Geometry check sheet. Reference: the model listing, model coordinates, mm. A direction names the side the tool comes from. Round coordinates to 2 decimals unless told otherwise and drop trailing zeros. Write each loop counter-clockwise with the first axis right and the second up, starting at its lowest first coordinate (ties: lowest second). Pieces come first, ordered by that corner, then holes. Notation, with made-up numbers: M 25,0.5 L 71,0.5 A14 ccw 71,25.5 Z; hole C 35.5,-31.75 d4. An arc over 180 degrees is marked long. Use a Markdown table: item, result.
```python
from build123d import *

# Parameters (mm, degrees)
EXTRUDE_2_DEPTH                = 14
FORK_ABOVE_MOUNTING_FOOT_DEPTH = 5
SKETCH_4_R                     = 2.6
OUTER_PIVOT_BORE_DEPTH         = 83.58934556
SKETCH_5_R                     = 2.6
UPPER_HINGE_BORE_DEPTH         = 83.58934556


with BuildPart() as part:
    # 草图1 → Extrude 2 (new body)
    with BuildSketch(Plane.XY):
        Polygon((-12, 60), (-25, 60), (-43, 42), (-55, 10.187667387), (-53, 5.924362391), (-20, 1.579829971), (-20, 9.579829971), (-44, 12.739489913), (-35, 36), (-12, 52), align=None)
    extrude(amount=EXTRUDE_2_DEPTH)

    # 草图3 → Fork_above_mounting_foot (cut, symmetric)
    with BuildSketch(Plane.XY.offset(7)):
        Polygon((5, 6.288517531), (-65, 15.504192362), (-65, 57), (5, 57), align=None)
    extrude(amount=FORK_ABOVE_MOUNTING_FOOT_DEPTH, both=True, mode=Mode.SUBTRACT)

    # 草图4 → Outer_pivot_bore (cut, through all)
    with BuildSketch(Plane.XY.offset(14)):
        with Locations((-40, 39)):
            Circle(SKETCH_4_R)
    extrude(amount=-OUTER_PIVOT_BORE_DEPTH, mode=Mode.SUBTRACT)

    # 草图5 → Upper_hinge_bore (cut, through all)
    with BuildSketch(Plane.XY.offset(14)):
        with Locations((-19, 55)):
            Circle(SKETCH_5_R)
    extrude(amount=-UPPER_HINGE_BORE_DEPTH, mode=Mode.SUBTRACT)


solid = part.part
```
Item 1: Cross-section at D-D, the plane y = 30. Record the cut outline in (x, z), and give its area (3 significant figures).
Outcome:
| item | result |
|---|---|
| outline | M -47.53,0 L -37.32,0 L -37.32,2 L -47.53,2 Z; M -47.53,12 L -37.32,12 L -37.32,14 L -47.53,14 Z |
| area | 40.8 mm2 |
Item 2: Access from +Z, -Z, +X, -X, +Y, -Y to the whole of each face (thin tool, end or side, straight path). Record for faces 4 (the face through (-19.338, 57.578, 7.098)), 5 (the face through (-24, 57, 7)), 6 (the face through (-39.56, 24.21, 12.99)), 7 (the face through (-15, 57, 7)), 8 (the face through (-20, 6, 7)).
Outcome:
| item | result |
|---|---|
| face 4 | +Z, -Z |
| face 5 | +X, -X |
| face 6 | +Z, -Z, +X |
| face 7 | +X, -X, -Y |
| face 8 | +Z, -Z, +X, -Y |
Item 3: Go/stop test with flat-tipped pins: pin 1 (1.6 mm diameter, centred on x = -15.5, z = 8, fed in from -Y); pin 2 (6 mm diameter, centred on x = -36.5, z = 10, fed in from -Y); pin 3 (3 mm diameter, centred on y = 36, z = 11.5, fed in from -X). Record where each tip stops, or that it passes through.
Outcome:
| item | result |
|---|---|
| pin 1 | stops at y = 57 |
| pin 2 | stops at y = 3.36 |
| pin 3 | stops at x = -45.8 |
Item 4: Cross-section at A-A, the plane y = 55. Record the cut outline in (x, z).
Outcome:
| item | result |
|---|---|
| outline | M -30,0 L -21.6,0 L -21.6,2 L -30,2 Z; M -30,12 L -21.6,12 L -21.6,14 L -30,14 Z; M -16.4,0 L -12,0 L -12,2 L -16.4,2 Z; M -16.4,12 L -12,12 L -12,14 L -16.4,14 Z |
Item 5: Cross-section at C-C, the plane x = -38.5. Record the cut outline in (y, z), and give its area (3 significant figures).
Outcome:
| item | result |
|---|---|
| outline | M 4.02,0 L 12.02,0 L 12.02,14 L 4.02,14 Z; M 26.95,0 L 36.88,0 L 36.88,2 L 26.95,2 Z; M 26.95,12 L 36.88,12 L 36.88,14 L 26.95,14 Z; M 41.12,0 L 46.5,0 L 46.5,2 L 41.12,2 Z; M 41.12,12 L 46.5,12 L 46.5,14 L 41.12,14 Z |
| area | 173 mm2 |
Item 6: Mould release check, pull along Y, two halves, no side actions. Record for faces 1 (the face through (-23.66, 43.89, 0.99)), 2 (the face through (-54.014, 8.086, 6.902)), 3 (the face through (-50.305, 22.633, 12.153)): +Y half, -Y half, draft (parallel to the pull), parting line (faces both ways), or undercut.
Outcome:
| item | result |
|---|---|
| face 1 | undercut |
| face 2 | -Y half |
| face 3 | +Y half |
Item 7: Material ranges on line 1 along Z through (x, y) = (-46, 33.5); line 2 along Y through (x, z) = (-26.5, 13.75); line 3 along Y through (x, z) = (-19, 4.5), recorded low to high. Write a range as from..to.
Outcome:
| item | result |
|---|---|
| line 1 | z = 0..2, 12..14 |
| line 2 | y = 2.44..10.44, 41.91..58.5 |
| line 3 | y = 57.6..60 |
Item 8: Cross-section at B-B, the plane z = 10.25. Record the cut outline in (x, y), and give its area (3 significant figures).
Outcome:
| item | result |
|---|---|
| outline | M -55,10.19 L -53,5.92 L -20,1.58 L -20,9.58 L -53.56,14 Z; M -28,57 L -20.66,57 A2.6 cw -17.34,57 L -12,57 L -12,60 L -25,60 Z |
| area | 315 mm2 |
